Autodesk Fusion 360 part; units mm, degrees
sketch "Sorted Smarties Collector" plane through (0, 0, 0) normal (0, 1, 0) x (1, 0, 0)
  line L0 (0, 0) -> (268, 0)
  line L1 (268, 0) -> (268, -262)
  line L2 (268, -262) -> (0, -262)
  line L3 (0, -262) -> (0, 0)
  dimension "d1" = 268
  dimension "d41" = 262
extrude "Extrude1" add sketch "Sorted Smarties Collector" along normal blind 3
sketch "Smartie Collectors" plane through (0, 3, 0) normal (0, 1, 0) x (-1, 0, 0)
  line L0 (0, 262) -> (-268, 262)
  line L1 (-268, 262) -> (-268, 0)
  line L2 (-268, 0) -> (0, 0)
  line L3 (0, 0) -> (0, 262)
  line L4 (-265, 259) -> (-201.75, 259)
  line L5 (-201.75, 259) -> (-201.75, 142.5)
  line L6 (-201.75, 142.5) -> (-265, 142.5)
  line L7 (-265, 142.5) -> (-265, 259)
  line L8 (-198.75, 259) -> (-135.5, 259)
  line L9 (-135.5, 259) -> (-135.5, 142.5)
  line L10 (-135.5, 142.5) -> (-198.75, 142.5)
  line L11 (-198.75, 142.5) -> (-198.75, 259)
  line L12 (-132.5, 259) -> (-69.25, 259)
  line L13 (-69.25, 259) -> (-69.25, 142.5)
  line L14 (-69.25, 142.5) -> (-132.5, 142.5)
  line L15 (-132.5, 142.5) -> (-132.5, 259)
  line L16 (-66.25, 259) -> (-3, 259)
  line L17 (-3, 259) -> (-3, 142.5)
  line L18 (-3, 142.5) -> (-66.25, 142.5)
  line L19 (-66.25, 142.5) -> (-66.25, 259)
  line L20 (-265, 139.5) -> (-201.75, 139.5)
  line L21 (-201.75, 139.5) -> (-201.75, 23)
  line L22 (-201.75, 23) -> (-265, 23)
  line L23 (-265, 23) -> (-265, 139.5)
  line L24 (-198.75, 139.5) -> (-135.5, 139.5)
  line L25 (-135.5, 139.5) -> (-135.5, 23)
  line L26 (-135.5, 23) -> (-198.75, 23)
  line L27 (-198.75, 23) -> (-198.75, 139.5)
  line L28 (-132.5, 139.5) -> (-69.25, 139.5)
  line L29 (-69.25, 139.5) -> (-69.25, 23)
  line L30 (-69.25, 23) -> (-132.5, 23)
  line L31 (-132.5, 23) -> (-132.5, 139.5)
  line L32 (-66.25, 139.5) -> (-3, 139.5)
  line L33 (-3, 139.5) -> (-3, 23)
  line L34 (-3, 23) -> (-66.25, 23)
  line L35 (-66.25, 23) -> (-66.25, 139.5)
  line L36 (-265, 0) -> (-3, 0)
  line L37 (-3, 0) -> (-3, 20)
  line L38 (-3, 20) -> (-265, 20)
  line L39 (-265, 20) -> (-265, 0)
  dimension "d51" = 3
  dimension "d52" = 3
  dimension "d53" = 3
  dimension "d54" = 20
  dimension "d55" = 3
  dimension "d56" = 3
  dimension "d57" = 3
  dimension "d58" = 3
  dimension "d59" = 3
  dimension "d60" = 116.5
  dimension "d61" = 116.5
  dimension "d62" = 63.25
  dimension "d63" = 63.25
  dimension "d64" = 63.25
  dimension "d65" = 63.25
extrude "Extrude2" add sketch "Smartie Collectors" along normal blind 69 contours L0 L1 L2 L3 L37 L38 L39
sketch "Front Panel" plane through (268, 0, 0) normal (1, 0, 0) x (0, 1, 0)
  line L0 (0, 262) -> (0, 0)
  line L1 (0, 0) -> (72, 0)
  line L2 (72, 0) -> (72, 262)
  line L3 (72, 262) -> (0, 262)
  line L4 (72, 262) -> (69, 262)
  line L5 (69, 262) -> (69, 0)
  line L6 (69, 0) -> (72, 0)
  line L7 (72, 0) -> (72, 262)
  dimension "d66" = 3
extrude "Extrude3" add sketch "Front Panel" against normal blind 268 contours L1 L2 L3 L4 L5 L6 L7
sketch "Front Openings" plane through (0, 72, 0) normal (0, 1, 0) x (-1, 0, 0)
  line L0 (-268, 0) -> (0, 0)
  line L1 (0, 0) -> (0, 262)
  line L2 (0, 262) -> (-268, 262)
  line L3 (-268, 262) -> (-268, 0)
  line L4 (0, 262) -> (-268, 262)
  line L5 (-198.75, 259) -> (-135.5, 259)
  line L6 (-265, 259) -> (-201.75, 259)
  line L7 (-201.75, 142.5) -> (-265, 142.5)
  line L8 (-265, 139.5) -> (-201.75, 139.5)
  line L9 (-201.75, 23) -> (-265, 23)
  line L10 (-135.5, 23) -> (-198.75, 23)
  line L11 (-69.25, 23) -> (-132.5, 23)
  line L12 (-3, 23) -> (-66.25, 23)
  line L13 (-132.5, 139.5) -> (-69.25, 139.5)
  line L14 (-198.75, 139.5) -> (-135.5, 139.5)
  line L15 (-135.5, 142.5) -> (-198.75, 142.5)
  line L16 (-69.25, 142.5) -> (-132.5, 142.5)
  line L17 (-3, 142.5) -> (-66.25, 142.5)
  line L18 (-66.25, 139.5) -> (-3, 139.5)
  line L19 (-132.5, 259) -> (-69.25, 259)
  line L20 (-66.25, 259) -> (-3, 259)
  line L21 (-3, 20) -> (-265, 20)
  line L22 (-3, 0) -> (-3, 20)
  line L23 (-265, 20) -> (-265, 0)
  line L24 (-265, 23) -> (-265, 139.5)
  line L25 (-201.75, 139.5) -> (-201.75, 23)
  line L26 (-198.75, 23) -> (-198.75, 139.5)
  line L27 (-135.5, 139.5) -> (-135.5, 23)
  line L28 (-132.5, 23) -> (-132.5, 139.5)
  line L29 (-69.25, 139.5) -> (-69.25, 23)
  line L30 (-66.25, 23) -> (-66.25, 139.5)
  line L31 (-3, 139.5) -> (-3, 23)
  line L32 (-265, 142.5) -> (-265, 259)
  line L33 (-201.75, 259) -> (-201.75, 142.5)
  line L34 (-198.75, 142.5) -> (-198.75, 259)
  line L35 (-135.5, 259) -> (-135.5, 142.5)
  line L36 (-132.5, 142.5) -> (-132.5, 259)
  line L37 (-69.25, 259) -> (-69.25, 142.5)
  line L38 (-66.25, 142.5) -> (-66.25, 259)
  line L39 (-3, 259) -> (-3, 142.5)
  line L40 (-265, 259) -> (-201.75, 259)
  line L41 (-201.75, 259) -> (-201.75, 181.3333)
  line L42 (-201.75, 181.3333) -> (-265, 181.3333)
  line L43 (-265, 181.3333) -> (-265, 259)
  line L44 (-198.75, 259) -> (-135.5, 259)
  line L45 (-135.5, 259) -> (-135.5, 181.3333)
  line L46 (-135.5, 181.3333) -> (-198.75, 181.3333)
  line L47 (-198.75, 181.3333) -> (-198.75, 259)
  line L48 (-132.5, 259) -> (-69.25, 259)
  line L49 (-69.25, 259) -> (-69.25, 181.3333)
  line L50 (-69.25, 181.3333) -> (-132.5, 181.3333)
  line L51 (-132.5, 181.3333) -> (-132.5, 259)
  line L52 (-66.25, 259) -> (-3, 259)
  line L53 (-3, 259) -> (-3, 181.3333)
  line L54 (-3, 181.3333) -> (-66.25, 181.3333)
  line L55 (-66.25, 181.3333) -> (-66.25, 259)
  line L56 (-265, 139.5) -> (-201.75, 139.5)
  line L57 (-201.75, 139.5) -> (-201.75, 61.8333)
  line L58 (-201.75, 61.8333) -> (-265, 61.8333)
  line L59 (-265, 61.8333) -> (-265, 139.5)
  line L60 (-198.75, 139.5) -> (-135.5, 139.5)
  line L61 (-135.5, 139.5) -> (-135.5, 61.8333)
  line L62 (-135.5, 61.8333) -> (-198.75, 61.8333)
  line L63 (-198.75, 61.8333) -> (-198.75, 139.5)
  line L64 (-132.5, 139.5) -> (-69.25, 139.5)
  line L65 (-69.25, 139.5) -> (-69.25, 61.8333)
  line L66 (-69.25, 61.8333) -> (-132.5, 61.8333)
  line L67 (-132.5, 61.8333) -> (-132.5, 139.5)
  line L68 (-66.25, 139.5) -> (-3, 139.5)
  line L69 (-3, 139.5) -> (-3, 61.8333)
  line L70 (-3, 61.8333) -> (-66.25, 61.8333)
  line L71 (-66.25, 61.8333) -> (-66.25, 139.5)
  line L72 (-3, 20) -> (-3, 0)
  line L73 (-3, 0) -> (-265, 0)
  line L74 (-265, 0) -> (-265, 20)
  dimension "d72" = 77.6667
  dimension "d73" = 77.6667
extrude "Extrude4" cut sketch "Front Openings" against normal blind 3 contours L5 L34 L35 L44 L45 L46 L47 | L6 L32 L33 L40 L41 L42 L43 | L8 L24 L25 L56 L57 L58 L59 | L14 L26 L27 L60 L61 L62 L63 | L13 L28 L29 L64 L65 L66 L67 | L18 L30 L31 L68 L69 L70 L71 | L19 L36 L37 L48 L49 L50 L51 | L20 L38 L39 L52 L53 L54 L55
sketch "Slide Handle" plane through (0, 0, 0) normal (0, -1, 0) x (1, 0, 0)
  line L0 (0, 262) -> (0, 0)
  line L1 (0, 0) -> (268, 0)
  line L2 (268, 0) -> (268, 262)
  line L3 (3, 20) -> (265, 20)
  line L4 (3, 0) -> (3, 20)
  line L5 (265, 20) -> (265, 0)
  line L6 (265, 0) -> (3, 0)
  line L7 (268, 262) -> (268, 0)
  line L8 (0, 0) -> (0, 262)
  line L9 (0, 262) -> (268, 262)
  line L10 (268, 0) -> (0, 0)
  line L11 (26, 0) -> (242, 0)
  line L12 (242, 0) -> (242, 20)
  line L13 (242, 20) -> (26, 20)
  line L14 (26, 20) -> (26, 0)
  circle A0 centre (26, 0) radius 20
  circle A1 centre (242, 0) radius 20
  point P0 (268, 0)
  dimension "d77" = 20
  dimension "d78" = 40
  dimension "d79" = 40
  dimension "d80" = 26
  dimension "d81" = 26
extrude "Extrude5" cut sketch "Slide Handle" against normal blind 72 contours L1 L6 L10 L14 A0 | L1 L6 L10 L11 L14 A0 | L1 L3 L6 L10 L11 L13 A0 A1 | L1 L6 L10 L12 A1 | L1 L6 L10 L11 L12 A1
equation "d1 = width"
equation "polycarbonateThickness = 3 mm"
equation "d3 = polycarbonateThickness"
equation "collectorWidth = ( width - 5 * polycarbonateThickness ) / 4"
equation "d37 = collectorLength - polycarbonateThickness"
equation "collectorHeight = ( height - 3 * polycarbonateThickness - bottomHeight ) / 2"
equation "height = 264 mm - tolerance"
equation "d41 = height"
equation "bottomHeight = 20 mm"
equation "d51 = polycarbonateThickness"
equation "d52 = polycarbonateThickness"
equation "d53 = polycarbonateThickness"
equation "d54 = bottomHeight"
equation "d55 = polycarbonateThickness"
equation "d56 = polycarbonateThickness"
equation "d57 = polycarbonateThickness"
equation "d58 = polycarbonateThickness"
equation "d59 = polycarbonateThickness"
equation "d60 = collectorHeight"
equation "d62 = collectorWidth"
equation "d63 = collectorWidth"
equation "d64 = collectorWidth"
equation "d66 = polycarbonateThickness"
equation "openingHeight = collectorHeight * 2 / 3"
equation "d72 = openingHeight"
equation "d73 = openingHeight"
equation "collectorLength = 72 mm"
equation "d80 = 2 * polycarbonateThickness + 20 mm"
equation "d81 = 2 * polycarbonateThickness + 20 mm"
equation "tolerance = 2 mm"
equation "width = 270 mm - tolerance"
The listing builds one solid part. Answer for the finished solid, in the listing's coordinates (mm). A direction names the side the tool comes from. Give positions to 0.01 mm unless a question says otherwise; leave off trailing zeros. Loops run counter-clockwise (first coordinate to the right, second up) from the corner with the lowest first, then second, coordinate; pieces in that order, holes last. Notation, with made-up numbers: (-31, -28.75) - (-19, -28.75) arc R31 cw to (-19, 0.25) - close; hole circle Ø10 at (50, 53.5). An arc over 180 degrees is marked (long way). Return JSON: item names as keys, results as strings. Group by question number.
1. Determine the mould class of faces 5 (the flat face through (135.5, 38, 202)), 6 (the flat face through (168, 38, 139.5)), 7 (the flat face through (3, 38, 202)) for opening direction Y: pulls with the +Y half, pulls with the -Y half, needs draft (parallel to the pull), parting line crosses it, or undercut.
2. Find section C-C (y = 61). State how many separate pieces and enclosed holes the cut face has, then the cut area to 3 significant figures.
3. Find section A-A (z = 244). Write down the section's boundary in (x, y).
4. Find section B-B (x = 146.5). Write down the section's boundary in (y, z), then the cut area to 3 significant figures.
5. Straight lines are drawn through the part: line 1 (X direction, y = 15.5, z = 114); line 2 (Z direction, x = 111.5, y = 13); line 3 (Y direction, x = 212, z = 36.5). For each, find the intervals that lie inside material, in ascending order. Write a range as [from, to].
6. Which of the six approach directions +Z, -Z, +X, -X, +Y, -Y give full straight-line access (tool end or side, diameter ignored) to faces 1 (the flat face through (132.5, 38, 80)), 2 (the flat face through (260, 3, 13)), 3 (the flat face through (234, 38, 259)), 4 (the cylindrical face through (12.014, 70.479, 14.297))?
7. Given pin 1 Ø3 at (x, y) = (119.5, 54.5) entering from -Z; pin 2 Ø8 at (x, z) = (172.5, 75.5) entering from +Y, each flat-ended and moving along its own axis, determine where each tip first touches the part or whether it passes through.
Verdict:
{
 "1": {"face 5": "undercut", "face 6": "needs draft", "face 7": "undercut"},
 "2": {"separate pieces": "1", "enclosed holes": "8", "area": "6,030 mm^2"},
 "3": {"outline": "(0, 0) - (268, 0) - (268, 72) - (265, 72) - (265, 3) - (201.75, 3) - (201.75, 72) - (198.75, 72) - (198.75, 3) - (135.5, 3) - (135.5, 72) - (132.5, 72) - (132.5, 3) - (69.25, 3) - (69.25, 72) - (66.25, 72) - (66.25, 3) - (3, 3) - (3, 72) - (0, 72) - close"},
 "4": {"outline": "(0, 20) - (72, 20) - (72, 61.83) - (69, 61.83) - (69, 23) - (3, 23) - (3, 139.5) - (72, 139.5) - (72, 181.33) - (69, 181.33) - (69, 142.5) - (3, 142.5) - (3, 259) - (72, 259) - (72, 262) - (0, 262) - close", "area": "1,580 mm^2"},
 "5": {"line 1": "x = [0, 3], [66.25, 69.25], [132.5, 135.5], [198.75, 201.75], [265, 268]", "line 2": "z = [20, 23], [139.5, 142.5], [259, 262]", "line 3": "y = [0, 3], [69, 72]"},
 "6": {"face 1": "none", "face 2": "-Z", "face 3": "+Y", "face 4": "-Z, +Y, -Y"},
 "7": {"pin 1": "stops at z = 20", "pin 2": "stops at y = 3"}
}
